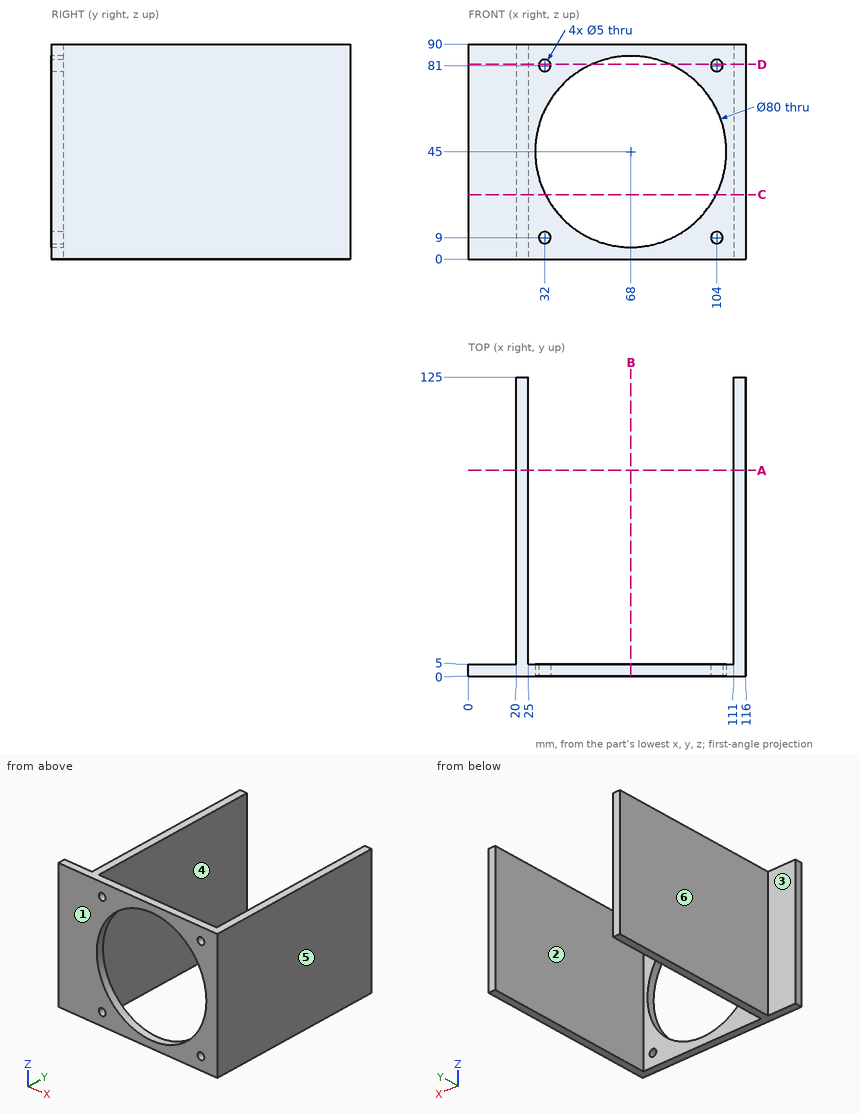
The drawing under review shows one solid part. Ordinate dimensions are in mm from its lowest x, y, z. A direction names the side the tool comes from. Round coordinates to 2 decimals unless told otherwise and drop trailing zeros. Write each loop counter-clockwise with the first axis right and the second up, starting at its lowest first coordinate (ties: lowest second). Pieces come first, ordered by that corner, then holes. Notation, with made-up numbers: (27, 53) -> (69, 53) arc R20 ccw to (69, 80) -> close; hole circle Ø2 at (71.5, -33). An arc over 180 degrees is marked (long way). Put each result on its own line as item: value.
Q1. Consider section C-C on z = 27. State the section outline as (x, y) points, and give its area (3 significant figures).
Determined:
outline: (0, 0) -> (32.28, 0) -> (32.28, 5) -> (25, 5) -> (25, 125) -> (20, 125) -> (20, 5) -> (0, 5) -> close; (103.72, 0) -> (116, 0) -> (116, 125) -> (111, 125) -> (111, 5) -> (103.72, 5) -> close
area: 1,420 mm^2
Q2. Clearance check with flat-ended pins moving along their axes: pin 1 Ø3 at (y, z) = (43, 24) entering from -X; pin 2 Ø22 at (x, z) = (8, 61.5) entering from +Y; pin 3 Ø12 at (x, z) = (42.5, 26.5) entering from -Y. State where each tip first meets the part, or that it passes through.
Determined:
pin 1: stops at x = 20
pin 2: stops at y = 5
pin 3: passes through
Q3. Consider section B-B on x = 68. State the section outline as (y, z) points.
Determined:
outline: (0, 0) -> (5, 0) -> (5, 5) -> (0, 5) -> close; (0, 85) -> (5, 85) -> (5, 90) -> (0, 90) -> close
Q4. Consider section A-A on y = 86. State the section outline as (x, z) points, and give its area (3 significant figures).
Determined:
outline: (20, 0) -> (25, 0) -> (25, 90) -> (20, 90) -> close; (111, 0) -> (116, 0) -> (116, 90) -> (111, 90) -> close
area: 900 mm^2
Q5. The part is to be moulded in two halves that separate along X. For the marked faces 3, 4, 5 and 6, say which applies: released by +X, released by -X, zero draft, split by the parting line, or undercut.
Determined:
face 3: zero draft
face 4: undercut
face 5: released by +X
face 6: released by -X
Q6. To check wall thickness, follow L1, parallel to X at y = 64.5, z = 74.5; L2, parallel to X at y = 2, z = 81; L3, parallel to Y at x = 10, z = 79. State the ranges of each line that lie inside material, in increasing order. Write a range as [from, to].
Determined:
L1: x = [20, 25], [111, 116]
L2: x = [0, 29.5], [34.5, 50.56], [85.44, 101.5], [106.5, 116]
L3: y = [0, 5]
Q7. Machinability: for the marked faces 1 and 2, which of the approach directions +Z, -Z, +X, -X, +Y, -Y give a long, thin tool a straight path to every point of the face, cutting with its end or side? Answer none if there is none.
Determined:
face 1: +Z, -Z, +X, -X, -Y
face 2: +Z, -Z, +Y
Q8. Consider section D-D on z = 81.5. State the section outline as (x, y) points, and give its area (3 significant figures).
Determined:
outline: (0, 0) -> (29.55, 0) -> (29.55, 5) -> (25, 5) -> (25, 125) -> (20, 125) -> (20, 5) -> (0, 5) -> close; (34.45, 0) -> (51.64, 0) -> (51.64, 5) -> (34.45, 5) -> close; (84.36, 0) -> (101.55, 0) -> (101.55, 5) -> (84.36, 5) -> close; (106.45, 0) -> (116, 0) -> (116, 125) -> (111, 125) -> (111, 5) -> (106.45, 5) -> close
area: 1,570 mm^2
